Autodesk Inventor part; units mm, degrees
ref_plane "Work Plane1" through (0, 0, 5) normal (0, 0, 1) x (1, 0, 0)
ref_plane "YZ Plane" through (0, 0, 0) normal (1, 0, 0) x (0, 1, 0)
ref_plane "XZ Plane" through (0, 0, 0) normal (0, 1, 0) x (-1, 0, 0)
sketch "Sketch1" plane through (0, 0, 0) normal (0, 0, 1) x (1, 0, 0)
  line L0 (14.6962, 12.74) -> (14.6962, 0) construction
  line L1 (10.61, 12.2) -> (1.53, 12.2)
  arc A0 (1.53, 12.2) -> (0, 10.67) centre (1.53, 10.67) ccw
  line L2 (0, 10.67) -> (0, 1.53)
  arc A1 (0, 1.53) -> (1.53, 0) centre (1.53, 1.53) ccw
  line L3 (1.53, 0) -> (10.61, 0)
  arc A2 (10.61, 0) -> (12.14, 1.53) centre (10.61, 1.53) ccw
  arc A3 (12.14, 10.67) -> (10.61, 12.2) centre (10.61, 10.67) ccw
  line L4 (12.14, 10.67) -> (12.14, 1.53)
  point P0 (0, 0)
  point P1 (0, 0)
  dimension "d10" = 12.74
ref_plane "Work Plane1" through (0, 0, 5) normal (0, 0, 1) x (1, 0, 0)
sketch "Sketch2" plane through (0, 0, 5) normal (0, 0, 1) x (1, 0, 0)
  line L0 (10.88, 12.74) -> (1.8, 12.74)
  line L1 (10.88, 12.74) -> (1.8, 12.74)
  arc A0 (1.8, 12.74) -> (0, 10.94) centre (1.8, 10.94) ccw
  line L2 (0, 10.94) -> (0, 1.8)
  arc A1 (0, 1.8) -> (1.8, 0) centre (1.8, 1.8) ccw
  line L3 (1.8, 0) -> (10.88, 0)
  arc A2 (10.88, 0) -> (12.68, 1.8) centre (10.88, 1.8) ccw
  line L4 (12.68, 1.8) -> (12.68, 10.94)
  arc A3 (12.68, 10.94) -> (10.88, 12.74) centre (10.88, 10.94) ccw
  circle A4 centre (6.34, 6.37) radius 2.8
  line L5 (5.665, 8.395) -> (7.015, 8.395)
  line L6 (7.015, 4.345) -> (5.665, 4.345)
  line L7 (5.665, 4.345) -> (7.015, 8.395) construction
  line L8 (5.665, 8.395) -> (7.015, 4.345) construction
  line L9 (8.365, 5.695) -> (8.365, 7.045)
  line L10 (4.315, 7.045) -> (4.315, 5.695)
  line L11 (4.315, 5.695) -> (8.365, 7.045) construction
  line L12 (8.365, 5.695) -> (4.315, 7.045) construction
  line L13 (4.315, 5.695) -> (5.665, 5.695)
  line L14 (7.015, 5.695) -> (8.365, 5.695)
  line L15 (5.665, 4.345) -> (5.665, 5.695)
  line L16 (5.665, 7.045) -> (5.665, 8.395)
  line L17 (8.365, 7.045) -> (7.015, 7.045)
  line L18 (5.665, 7.045) -> (4.315, 7.045)
  line L19 (7.015, 8.395) -> (7.015, 7.045)
  line L20 (7.015, 5.695) -> (7.015, 4.345)
  point P0 (0, 0)
  dimension "d3" = 5.6
  dimension "d4" = 4.05
  dimension "d5" = 1.35
  dimension "d6" = 4.05
  dimension "d7" = 1.35
extrude "Extrusion3" add sketch "Sketch1" along normal blind 5
sketch "Sketch3" plane through (0, 0, 5) normal (0, 0, 1) x (1, 0, 0)
  line L0 (10.61, 12.47) -> (1.53, 12.47)
  line L1 (10.61, 12.47) -> (1.53, 12.47)
  arc A0 (1.53, 12.47) -> (-0.27, 10.67) centre (1.53, 10.67) ccw
  line L2 (-0.27, 10.67) -> (-0.27, 1.53)
  arc A1 (-0.27, 1.53) -> (1.53, -0.27) centre (1.53, 1.53) ccw
  line L3 (1.53, -0.27) -> (10.61, -0.27)
  arc A2 (10.61, -0.27) -> (12.41, 1.53) centre (10.61, 1.53) ccw
  line L4 (12.41, 1.53) -> (12.41, 10.67)
  arc A3 (12.41, 10.67) -> (10.61, 12.47) centre (10.61, 10.67) ccw
  circle A4 centre (6.07, 6.1) radius 2.8
  line L5 (5.395, 8.125) -> (6.745, 8.125)
  line L6 (6.745, 4.075) -> (5.395, 4.075)
  line L7 (5.395, 4.075) -> (6.745, 8.125) construction
  line L8 (5.395, 8.125) -> (6.745, 4.075) construction
  line L9 (8.095, 5.425) -> (8.095, 6.775)
  line L10 (4.045, 6.775) -> (4.045, 5.425)
  line L11 (4.045, 5.425) -> (8.095, 6.775) construction
  line L12 (8.095, 5.425) -> (4.045, 6.775) construction
  line L13 (4.045, 5.425) -> (5.395, 5.425)
  line L14 (6.745, 5.425) -> (8.095, 5.425)
  line L15 (5.395, 4.075) -> (5.395, 5.425)
  line L16 (5.395, 6.775) -> (5.395, 8.125)
  line L17 (8.095, 6.775) -> (6.745, 6.775)
  line L18 (5.395, 6.775) -> (4.045, 6.775)
  line L19 (6.745, 8.125) -> (6.745, 6.775)
  line L20 (6.745, 5.425) -> (6.745, 4.075)
  line L21 (10.61, 12.2) -> (1.53, 12.2)
  line L22 (0, 10.67) -> (0, 1.53)
  point P0 (0, 0)
  point P1 (-0.27, -0.27)
  point P2 (6.07, 12.2)
  point P3 (0, 6.1)
  point P4 (6.07, 6.1)
  dimension "d14" = 5.6
  dimension "d15" = 4.05
  dimension "d16" = 1.35
  dimension "d17" = 4.05
  dimension "d18" = 1.35
extrude "Extrusion4" add sketch "Sketch3" along normal blind 4.8 contours A4
sketch "Sketch4" plane through (0, 0, 0) normal (0, 0, -1) x (-1, 0, 0)
  line L0 (-1.53, 0) -> (-10.61, 0)
  line L1 (-11.7223, 9.7129) -> (-0.4177, 9.7129) construction
  line L2 (-0.4177, 9.7129) -> (-0.4177, 6.84) construction
  line L3 (-0.4177, 6.84) -> (-11.7223, 6.84) construction
  line L4 (-11.7223, 6.84) -> (-11.7223, 9.7129) construction
  line L5 (-7.4059, 5.3753) -> (-4.7341, 5.3753) construction
  line L6 (-4.7341, 5.3753) -> (-4.7341, 2.266) construction
  line L7 (-4.7341, 2.266) -> (-7.4059, 2.266) construction
  line L8 (-7.4059, 2.266) -> (-7.4059, 5.3753) construction
  line L9 (-11.7333, 6.956) -> (-10.8209, 9.656)
  line L10 (-10.8209, 9.656) -> (-10.0813, 9.656)
  line L11 (-10.0813, 9.656) -> (-9.1689, 6.956)
  line L12 (-9.1689, 6.956) -> (-9.8669, 6.956)
  line L13 (-9.8669, 6.956) -> (-10.0354, 7.5074)
  line L14 (-10.0354, 7.5074) -> (-10.8843, 7.5074)
  line L15 (-10.8843, 7.5074) -> (-11.055, 6.956)
  line L16 (-11.055, 6.956) -> (-11.7333, 6.956)
  line L17 (-10.1842, 7.9975) -> (-10.4598, 8.8902)
  line L18 (-10.4598, 8.8902) -> (-10.7377, 7.9975)
  line L19 (-10.7377, 7.9975) -> (-10.1842, 7.9975)
  line L20 (-7.0991, 6.956) -> (-8.8998, 6.956)
  line L21 (-8.8998, 6.956) -> (-8.8998, 9.656)
  line L22 (-8.8998, 9.656) -> (-8.2215, 9.656)
  line L23 (-8.2215, 9.656) -> (-8.2215, 7.4702)
  line L24 (-8.2215, 7.4702) -> (-7.0991, 7.4702)
  line L25 (-7.0991, 7.4702) -> (-7.0991, 6.956)
  spline S0 degree 2 poles (-4.3181, 8.306) (-4.3181, 7.6496) (-5.0183, 6.8991) (-5.6265, 6.8991) knots 0 0 0 1 2 2 2
  spline S1 degree 2 poles (-5.6265, 6.8991) (-6.237, 6.8991) (-6.9328, 7.6584) (-6.9328, 8.306) knots 0 0 0 1 2 2 2
  spline S2 degree 2 poles (-6.9328, 8.306) (-6.9328, 8.9559) (-6.237, 9.7129) (-5.6265, 9.7129) knots 0 0 0 1 2 2 2
  spline S3 degree 2 poles (-5.6265, 9.7129) (-5.0183, 9.7129) (-4.3181, 8.9602) (-4.3181, 8.306) knots 0 0 0 1 2 2 2
  spline S4 degree 2 poles (-5.0183, 8.306) (-5.0183, 8.5489) (-5.1167, 8.888) (-5.2021, 8.9952) knots 0 0 0 1 2 2 2
  spline S5 degree 2 poles (-5.2021, 8.9952) (-5.2874, 9.1068) (-5.5062, 9.2031) (-5.6243, 9.2031) knots 0 0 0 1 2 2 2
  spline S6 degree 2 poles (-5.6243, 9.2031) (-5.7491, 9.2031) (-5.9525, 9.1134) (-6.0466, 8.9996) knots 0 0 0 1 2 2 2
  spline S7 degree 2 poles (-6.0466, 8.9996) (-6.1298, 8.8946) (-6.2326, 8.5467) (-6.2326, 8.306) knots 0 0 0 1 2 2 2
  spline S8 degree 2 poles (-6.2326, 8.306) (-6.2326, 8.0566) (-6.1342, 7.7284) (-6.0488, 7.6168) knots 0 0 0 1 2 2 2
  spline S9 degree 2 poles (-6.0488, 7.6168) (-5.9635, 7.5052) (-5.7425, 7.4089) (-5.6243, 7.4089) knots 0 0 0 1 2 2 2
  spline S10 degree 2 poles (-5.6243, 7.4089) (-5.504, 7.4089) (-5.2808, 7.5118) (-5.1999, 7.6212) knots 0 0 0 1 2 2 2
  spline S11 degree 2 poles (-5.1999, 7.6212) (-5.1124, 7.7393) (-5.0183, 8.0522) (-5.0183, 8.306) knots 0 0 0 1 2 2 2
  line L26 (-0.4344, 9.656) -> (-1.1171, 6.956)
  line L27 (-1.1171, 6.956) -> (-1.861, 6.956)
  line L28 (-1.861, 6.956) -> (-2.2942, 8.6255)
  line L29 (-2.2942, 8.6255) -> (-2.7121, 6.956)
  line L30 (-2.7121, 6.956) -> (-3.4582, 6.956)
  line L31 (-3.4582, 6.956) -> (-4.1409, 9.656)
  line L32 (-4.1409, 9.656) -> (-3.4363, 9.656)
  line L33 (-3.4363, 9.656) -> (-3.0644, 7.8487)
  line L34 (-3.0644, 7.8487) -> (-2.6136, 9.656)
  line L35 (-2.6136, 9.656) -> (-1.9397, 9.656)
  line L36 (-1.9397, 9.656) -> (-1.5109, 7.8465)
  line L37 (-1.5109, 7.8465) -> (-1.1214, 9.656)
  line L38 (-1.1214, 9.656) -> (-0.4344, 9.656)
  line L39 (-4.8552, 2.266) -> (-7.097, 2.266)
  line L40 (-7.097, 2.266) -> (-7.097, 2.7628)
  spline S12 degree 2 poles (-7.097, 2.7628) (-6.8127, 2.9902) (-6.3579, 3.3906) (-6.1874, 3.571) knots 0 0 0 1 2 2 2
  spline S13 degree 2 poles (-6.1874, 3.571) (-5.9625, 3.8058) (-5.7623, 4.1642) (-5.7623, 4.3521) knots 0 0 0 1 2 2 2
  spline S14 degree 2 poles (-5.7623, 4.3521) (-5.7623, 4.5646) (-6.0169, 4.792) (-6.2443, 4.792) knots 0 0 0 1 2 2 2
  spline S15 degree 2 poles (-6.2443, 4.792) (-6.3604, 4.792) (-6.568, 4.7352) (-6.6743, 4.6907) knots 0 0 0 1 2 2 2
  spline S16 degree 2 poles (-6.6743, 4.6907) (-6.7781, 4.6437) (-6.9264, 4.5448) (-6.9635, 4.5201) knots 0 0 0 1 2 2 2
  line L41 (-6.9635, 4.5201) -> (-7.0228, 4.5201)
  line L42 (-7.0228, 4.5201) -> (-7.0228, 5.185)
  spline S17 degree 2 poles (-7.0228, 5.185) (-6.8943, 5.2468) (-6.3456, 5.3753) (-6.091, 5.3753) knots 0 0 0 1 2 2 2
  spline S18 degree 2 poles (-6.091, 5.3753) (-5.5472, 5.3753) (-4.9887, 4.8909) (-4.9887, 4.4534) knots 0 0 0 1 2 2 2
  spline S19 degree 2 poles (-4.9887, 4.4534) (-4.9887, 4.184) (-5.2432, 3.6649) (-5.5374, 3.3684) knots 0 0 0 1 2 2 2
  spline S20 degree 2 poles (-5.5374, 3.3684) (-5.7227, 3.1854) (-6.0712, 2.9012) (-6.1479, 2.8419) knots 0 0 0 1 2 2 2
  line L43 (-6.1479, 2.8419) -> (-4.8552, 2.8419)
  line L44 (-4.8552, 2.8419) -> (-4.8552, 2.266)
  point P0 (0, 0)
  point P1 (-6.07, 2.266)
  point P2 (-6.07, 6.84)
  point P3 (-6.07, 6.84)
  point P4 (-6.07, 2.266)
extrude "Extrusion5" add sketch "Sketch4" along normal blind 0.9
properties part number "IPC ALOW 2 key"
Verification items for the finished model (mm, model axes). A direction names the side the tool comes from. Give positions to 0.01 mm unless a question says otherwise; leave off trailing zeros. Order: outer loops, then holes, each group sorted by start corner. A loop starts at its lowest first (then second) coordinate and runs counter-clockwise, first axis right, second up. Notation, with made-up numbers: M 72,-26 L 94,-26 A33 ccw 94,12 Z; hole C 22,69 d6. An arc over 180 degrees is marked long. Answer as a JSON object with one key per item and string values. Group by question number.
1) Scan lines: line 1 along Y through (x, z) = (6, 6.5) (3 decimals); line 2 along Z through (x, y) = (7, 1.5); line 3 along Z through (x, y) = (8.5, 8.5). Record each from-to range of solid material in increasing order. Write a range as [from, to].
2) Cross-section at D-D (y = 10). Enter the section's corners in (x, z).
3) Depth check by flat-ended pin: pin 1 Ø1.1 at (y, z) = (7.5, 8.5) entering from -X; pin 2 Ø0.7 at (y, z) = (6, 7.5) entering from +X; pin 3 Ø1.5 at (y, z) = (4.5, 8) entering from +X. Enter the tip coordinate at first touch or a pass-through.
4) Mould release check, pull along X, two halves, no side actions. Record for faces 5 (the face through (11.68, 11.764, 2.465)), 6 (the face through (7, 5, 9.8)), 7 (the face through (10.32, 8.44, -0.44)): released by +X, released by -X, zero draft, split by the parting line, or undercut.
5) Cross-section at A-A (z = 7.5). Enter the section's corners in (x, y) (3 decimals), then the cut area to 3 significant figures.
6) Cross-section at C-C (x = 8.5). Enter the section's corners in (y, z).
7) Cross-section at B-B (y = 6.1). Enter the section's corners in (x, z) (3 decimals).
8) Access from +Z, -Z, +X, -X, +Y, -Y to the whole of each face (thin tool, end or side, straight path). Record for faces 1 (the face through (6, 8, 0)), 2 (the face through (6, 4.075, 7)), 3 (the face through (6, 2.266, -0.4)), 4 (the face through (11.283, 8.287, -0.444)).
Result sheet:
{
 "1": {"line 1": "y = [3.301, 4.075], [8.125, 8.899]", "line 2": "z = [0, 5]", "line 3": "z = [-0.9, 5]"},
 "2": {"outline": "M 0,0 L 12.14,0 L 12.14,5 L 0,5 Z"},
 "3": {"pin 1": "stops at x = 3.4", "pin 2": "stops at x = 8.87", "pin 3": "stops at x = 8.74"},
 "4": {"face 5": "released by +X", "face 6": "zero draft", "face 7": "undercut"},
 "5": {"outline": "C 6.07,6.1 d5.6; hole M 4.045,5.425 L 5.395,5.425 L 5.395,4.075 L 6.745,4.075 L 6.745,5.425 L 8.095,5.425 L 8.095,6.775 L 6.745,6.775 L 6.745,8.125 L 5.395,8.125 L 5.395,6.775 L 4.045,6.775 Z", "area": "15.5 mm2"},
 "6": {"outline": "M 0,0 L 6.96,0 L 6.96,-0.9 L 9.66,-0.9 L 9.66,0 L 12.2,0 L 12.2,5 L 7.49,5 L 7.49,9.8 L 4.71,9.8 L 4.71,5 L 0,5 Z"},
 "7": {"outline": "M 0,0 L 12.14,0 L 12.14,5 L 8.87,5 L 8.87,9.8 L 8.095,9.8 L 8.095,5 L 4.045,5 L 4.045,9.8 L 3.27,9.8 L 3.27,5 L 0,5 Z"},
 "8": {"face 1": "-Z", "face 2": "+Z", "face 3": "-Z, +X, -X, -Y", "face 4": "-Z, +X, +Y"}
}
